from build123d import *

# Parameters (mm, degrees)
F1_DEPTH = 15
F2_DEPTH = 3
F3_R     = 1.49999


# Not quite as in the source:
# - a fillet or chamfer is up to 0.001 mm smaller than in the source, because OpenCascade refuses the exact size


with BuildPart() as f1:
    # F0 (on Top) → F1 (new body)
    with BuildSketch(Plane.XY):
        with BuildLine():
            ThreePointArc((-22.6053091109, -33), (-18.6519119069, 35.3851124376), (40, 0))
            ThreePointArc((40, 0), (35.3851124376, -18.6519119069), (22.6053091109, -33))
            Line((22.6053091109, -33), (27.5680975042, -33))
            ThreePointArc((27.5680975042, -33), (38.9514325326, -18.2149911792), (43, 0))
            ThreePointArc((43, 0), (-18.2149911792, 38.9514325326), (-27.5680975042, -33))
            Line((-27.5680975042, -33), (-22.6053091109, -33))
        make_face()
    extrude(amount=F1_DEPTH)

    # F0 (on Top) → F2 (join)
    with BuildSketch(Plane.XY):
        with BuildLine():
            ThreePointArc((22.6053091109, -33), (35.3851124376, -18.6519119069), (40, 0))
            ThreePointArc((40, 0), (-18.6519119069, 35.3851124376), (-22.6053091109, -33))
            Line((-22.6053091109, -33), (22.6053091109, -33))
        make_face()
    extrude(amount=F2_DEPTH)

    # F3 (radius 1.5 in the source; OpenCascade refuses exactly that, so slightly less here)
    f3_edges = [f1.edges().sort_by_distance(p)[0] for p in [
        (-22.605309, -33, 9),
        (22.605309, -33, 9),
        (-27.568098, -33, 7.5),
        (27.568098, -33, 7.5),
    ]]
    fillet(f3_edges, radius=F3_R)


solid = f1.part
Design review of the part built by this model. Coordinates are the model's own, in mm. A direction names the side the tool comes from. Give positions to 0.01 mm unless a question says otherwise; leave off trailing zeros. Loops run counter-clockwise (first coordinate to the right, second up) from the corner with the lowest first, then second, coordinate; pieces in that order, holes last. Notation, with made-up numbers: (72, -9) -> (119, -9) arc R32 cw to (119, 22) -> close; hole circle Ø2 at (86.5, 10). An arc over 180 degrees is marked (long way). One line per question, with ' | ' between items. Start each with the question number.
(1) We need section A-A (x = 0). State the section outline as (y, z) points, and give its area (3 significant figures).
(2) For faces 1 (the face through (-10, 39, 15)), 2 (the face through (25.62, -32.04, 9.08)), list the 3-axis set-ups (+Z, -Z, +X, -X, +Y, -Y) from which the entire face can be reached by the end or side of a thin tool; tool diameter is ignored.
(3) We need section C-C (y = 15). State the section outline as (x, z) points, and give its area (3 significant figures).
(4) Insertion check: P1, Ø8, axis at x = 32.5, z = 5.5, coming from the -Y side; P2, Ø3, axis at x = 20.5, z = 5, coming from the +Y side; P3, Ø2, axis at x = -3, y = -22.5, coming from the +Z side. Each pin has a flat end and moves straight along its axis. Give the tip position at first contact, or say it passes through.
(5) For line 1 (Y direction, x = 0, z = 5.5); line 2 (Z direction, x = -13, y = 0); line 3 (X direction, y = -3.5, z = 8), list the stretches that pass through material, from the lowest coordinate up.
(6) We need section D-D (x = 32). State the section outline as (y, z) points, and give its area (3 significant figures).
(7) Draft analysis for pull direction Y (two halves, no side actions). For faces 3 (the face through (-1, 6, 0)), 4 (the face through (-1, 4, 3)), 5 (the face through (1.464, 42.975, 7.395)), 6 (the face through (0, -33, 1)), state which applies: +Y half, -Y half, draft (parallel to the pull), parting line (faces both ways), or undercut.
The answers:
1) outline: (-33, 0) -> (43, 0) -> (43, 15) -> (40, 15) -> (40, 3) -> (-33, 3) -> close | area: 264 mm^2
2) face 1: +Z, +X, -X, +Y, -Y | face 2: +Z
3) outline: (-40.3, 0) -> (40.3, 0) -> (40.3, 15) -> (37.08, 15) -> (37.08, 3) -> (-37.08, 3) -> (-37.08, 15) -> (-40.3, 15) -> close | area: 319 mm^2
4) P1: stops at y = -32.2 | P2: stops at y = 38.57 | P3: stops at z = 3
5) line 1: y = 40 to 43 | line 2: z = 0 to 3 | line 3: x = -42.86 to -39.85, 39.85 to 42.86
6) outline: (-28.72, 0) -> (28.72, 0) -> (28.72, 15) -> (24, 15) -> (24, 3) -> (-24, 3) -> (-24, 15) -> (-28.72, 15) -> close | area: 286 mm^2
7) face 3: draft | face 4: undercut | face 5: parting line | face 6: -Y half
